CAD build for the part. Positions are in the model's coordinates, mm. A direction names the side the tool comes from. Give positions to 0.01 mm unless a question says otherwise; leave off trailing zeros. Write each loop counter-clockwise with the first axis right and the second up, starting at its lowest first coordinate (ties: lowest second). Pieces come first, ordered by that corner, then holes. Notation, with made-up numbers: (12, 31) - (24, 31) arc R20 ccw to (24, 64) - close; hole circle Ø6 at (-10.5, 73). An arc over 180 degrees is marked (long way). Answer as a JSON object with one key per item and string values.
from build123d import *

# Parameters (mm, degrees)
SKETCH1_W                                     = 80
SKETCH1_H                                     = 80
BOSS_EXTRUDE1_DEPTH                           = 23.7
CUT_EXTRUDE1_DEPTH                            = 1
SKETCH3_W                                     = 15
SKETCH3_H                                     = 15
CUT_EXTRUDE2_DEPTH                            = 95.785112281
SKETCH4_W                                     = 60
SKETCH4_H                                     = 13.7
CUT_EXTRUDE3_DEPTH                            = 114.918214427
SKETCH5_R                                     = 3
SKETCH5_R_2                                   = 2
CUT_EXTRUDE4_DEPTH                            = 114.918214427
CBORE_FOR_M5_HEX_SOCKET_HEAD_CAP1_D           = 5.5
CBORE_FOR_M5_HEX_SOCKET_HEAD_CAP1_CBORE_D     = 10
CBORE_FOR_M5_HEX_SOCKET_HEAD_CAP1_CBORE_DEPTH = 15
M3X0_5_TAPPED_HOLE1_D                         = 2.5
M2X0_4_TAPPED_HOLE1_REACH                     = 95.041
M2X0_4_TAPPED_HOLE1_BORE_R                    = 0.8


with BuildPart() as part:
    # Sketch1 → Boss-Extrude1 (new body)
    with BuildSketch(Plane(origin=(0, 0, 0), x_dir=(1, 0, 0), z_dir=(0, 1, 0))):
        with Locations((-37.560747664, 9.530373832)):
            Rectangle(SKETCH1_W, SKETCH1_H)
    extrude(amount=BOSS_EXTRUDE1_DEPTH)

    # Sketch2 → Cut-Extrude1 (cut)
    with BuildSketch(Plane(origin=(0, 23.7, 0), x_dir=(1, 0, 0), z_dir=(0, 1, 0))):
        Polygon((2.439252336, -28.669626168), (-22.560747664, -28.669626168), (-22.560747664, -18.669626168), (-32.560747664, -18.669626168), (-32.560747664, -28.669626168), (-67.560747664, -28.669626168), (-67.560747664, 47.730373832), (-32.560747664, 47.730373832), (-32.560747664, 37.730373832), (-22.560747664, 37.730373832), (-22.560747664, 47.730373832), (2.439252336, 47.730373832), align=None)
    extrude(amount=-CUT_EXTRUDE1_DEPTH, mode=Mode.SUBTRACT)

    # Sketch3 → Cut-Extrude2 (cut, through all)
    with BuildSketch(Plane(origin=(0, 22.7, 0), x_dir=(1, 0, 0), z_dir=(0, 1, 0))):
        with Locations((-55.060747664, -16.169626168)):
            Rectangle(SKETCH3_W, SKETCH3_H)
        with Locations((-55.060747664, 5.830373832)):
            Rectangle(SKETCH3_W, SKETCH3_H)
        with Locations((-55.060747664, 27.830373832)):
            Rectangle(SKETCH3_W, SKETCH3_H)
    extrude(amount=-CUT_EXTRUDE2_DEPTH, mode=Mode.SUBTRACT)

    # Sketch4 → Cut-Extrude3 (cut, through all)
    with BuildSketch(Plane.XY.offset(30.469626168)):
        with Locations((-47.560747664, 6.85)):
            Rectangle(SKETCH4_W, SKETCH4_H)
    extrude(amount=-CUT_EXTRUDE3_DEPTH, mode=Mode.SUBTRACT)

    # Sketch5 → Cut-Extrude4 (cut, through all)
    with BuildSketch(Plane.XY.offset(30.469626168)):
        with Locations((-66.560747664, 18.7)):
            Circle(SKETCH5_R)
        with Locations((-44.560747664, 18.7)):
            Circle(SKETCH5_R_2)
    extrude(amount=-CUT_EXTRUDE4_DEPTH, mode=Mode.SUBTRACT)

    # CBORE for M5 Hex Socket Head Cap1 (through all)
    with Locations(Plane(origin=(0, 22.7, 0), x_dir=(1, 0, 0), z_dir=(0, 1, 0))):
        with Locations((-7.560747664, -20.469626168), (-7.560747664, -0.469626168), (-7.560747664, 19.530373832), (-7.560747664, 39.530373832)):
            CounterBoreHole(CBORE_FOR_M5_HEX_SOCKET_HEAD_CAP1_D / 2, CBORE_FOR_M5_HEX_SOCKET_HEAD_CAP1_CBORE_D / 2, CBORE_FOR_M5_HEX_SOCKET_HEAD_CAP1_CBORE_DEPTH)

    # M3x0.5 Tapped Hole1 (through all)
    with Locations(Plane(origin=(0, 23.7, 0), x_dir=(1, 0, 0), z_dir=(0, 1, 0))):
        with Locations((-27.560747664, -23.669626168), (-27.560747664, 42.730373832), (-72.523263375, -23.669626168), (-72.523263375, 42.730373832)):
            Hole(M3X0_5_TAPPED_HOLE1_D / 2)

    # M2x0.4 Tapped Hole1 bore → M2x0.4 Tapped Hole1 (cut, up to next)
    with BuildSketch(Plane(origin=(0, 13.7, 0), x_dir=(-1, 0, 0), z_dir=(0, -1, 0)), mode=Mode.PRIVATE) as m2x0_4_tapped_hole1_sk1:
        with Locations((66.560747664, -15.469626168)):
            Circle(M2X0_4_TAPPED_HOLE1_BORE_R)
    m2x0_4_tapped_hole1_tool1 = extrude(m2x0_4_tapped_hole1_sk1.sketch, amount=-M2X0_4_TAPPED_HOLE1_REACH, mode=Mode.PRIVATE) & part.part
    # M2x0.4 Tapped Hole1 bore → M2x0.4 Tapped Hole1 (cut, up to next)
    with BuildSketch(Plane(origin=(0, 13.7, 0), x_dir=(-1, 0, 0), z_dir=(0, -1, 0)), mode=Mode.PRIVATE) as m2x0_4_tapped_hole1_sk2:
        with Locations((44.560747664, -15.469626168)):
            Circle(M2X0_4_TAPPED_HOLE1_BORE_R)
    m2x0_4_tapped_hole1_tool2 = extrude(m2x0_4_tapped_hole1_sk2.sketch, amount=-M2X0_4_TAPPED_HOLE1_REACH, mode=Mode.PRIVATE) & part.part
    # M2x0.4 Tapped Hole1 bore → M2x0.4 Tapped Hole1 (cut, up to next)
    with BuildSketch(Plane(origin=(0, 13.7, 0), x_dir=(-1, 0, 0), z_dir=(0, -1, 0)), mode=Mode.PRIVATE) as m2x0_4_tapped_hole1_sk3:
        with Locations((66.560747664, 34.530373832)):
            Circle(M2X0_4_TAPPED_HOLE1_BORE_R)
    m2x0_4_tapped_hole1_tool3 = extrude(m2x0_4_tapped_hole1_sk3.sketch, amount=-M2X0_4_TAPPED_HOLE1_REACH, mode=Mode.PRIVATE) & part.part
    # M2x0.4 Tapped Hole1 bore → M2x0.4 Tapped Hole1 (cut, up to next)
    with BuildSketch(Plane(origin=(0, 13.7, 0), x_dir=(-1, 0, 0), z_dir=(0, -1, 0)), mode=Mode.PRIVATE) as m2x0_4_tapped_hole1_sk4:
        with Locations((44.560747664, 34.530373832)):
            Circle(M2X0_4_TAPPED_HOLE1_BORE_R)
    m2x0_4_tapped_hole1_tool4 = extrude(m2x0_4_tapped_hole1_sk4.sketch, amount=-M2X0_4_TAPPED_HOLE1_REACH, mode=Mode.PRIVATE) & part.part
    add(m2x0_4_tapped_hole1_tool1.solids().sort_by_distance((-66.560748, 13.7, 15.469626))[0], mode=Mode.SUBTRACT)
    add(m2x0_4_tapped_hole1_tool2.solids().sort_by_distance((-44.560748, 13.7, 15.469626))[0], mode=Mode.SUBTRACT)
    add(m2x0_4_tapped_hole1_tool3.solids().sort_by_distance((-66.560748, 13.7, -34.530374))[0], mode=Mode.SUBTRACT)
    add(m2x0_4_tapped_hole1_tool4.solids().sort_by_distance((-44.560748, 13.7, -34.530374))[0], mode=Mode.SUBTRACT)


solid = part.part
Item 1: Probe line 1 (Z direction, x = -7.5, y = 14.25); line 2 (Z direction, x = -52, y = 19.5); line 3 (X direction, y = 17, z = -22). List the from-to ranges inside material, lowest first. Write a range as from..to.
Entries:
{"line 1": "-49.53..-44.53, -34.53..-24.53, -14.53..-4.53, 5.47..15.47, 25.47..30.47", "line 2": "-49.53..-35.33, -20.33..-13.33, 1.67..8.67, 23.67..30.47", "line 3": "-77.56..-69.03, -64.09..-62.56, -47.56..-45.61, -43.51..-11.91, -3.21..2.44"}
Item 2: Mould opens along Z. For faces 4 (the flat face through (-8, 0, -10)), 5 (the flat face through (-55, 18, -20.33)), 6 (the flat face through (-29, 14, 30.47)) say: +Z half, -Z half, draft (parallel to the pull), parting line (faces both ways), or undercut.
Entries:
{"face 4": "draft", "face 5": "undercut", "face 6": "+Z half"}
Item 3: Cut at C-C (x = -16.5). Give the cut face in (y, z).
Entries:
{"outline": "(0, -49.53) - (23.7, -49.53) - (23.7, -47.73) - (22.7, -47.73) - (22.7, 28.67) - (23.7, 28.67) - (23.7, 30.47) - (0, 30.47) - close"}
Item 4: Cut at B-B (y = 18.7). State how many separate pieces and enclosed holes the cut face has, and give its area (3 significant figures).
Entries:
{"separate pieces": "3", "enclosed holes": "11", "area": "4,590 mm2"}
Item 5: Which spindle directions (+Z, -Z, +X, -X, +Y, -Y) get a long thin tool onto all of the face, cutting with end or side? Do faces 1 (the flat face through (-47.561, 18, -6)), 2 (the flat face through (-41, 13.7, -9)), 3 (the flat face through (-5, 7.7, -17)). Say none if no direction does.
Entries:
{"face 1": "+Y, -Y", "face 2": "+Z, -Z, -X, -Y", "face 3": "+Y"}
Item 6: Flat gauge pins, fed straight in: P1, Ø5, axis at x = -6, z = -17, coming from the +Y side; P2, Ø8, axis at x = -7.56, z = -19.53, coming from the +Y side; P3, Ø0.8, axis at y = 23.5, z = 25.5, coming from the +X side; P4, Ø4.5, axis at x = -7.56, z = -19.53, coming from the -Y side. Where does each tip first touch, or does it go through?
Entries:
{"P1": "y = 22.7", "P2": "y = 7.7", "P3": "x = -22.56", "P4": "through"}
Item 7: Cut at D-D (y = 2.25). Give the cut face in (x, z).
Entries:
{"outline": "(-17.56, -49.53) - (2.44, -49.53) - (2.44, 30.47) - (-17.56, 30.47) - close; hole circle Ø5.5 at (-7.56, -39.53); hole circle Ø5.5 at (-7.56, -19.53); hole circle Ø5.5 at (-7.56, 0.47); hole circle Ø5.5 at (-7.56, 20.47)"}
Item 8: Cut at A-A (z = 12). Give the cut face in (x, y), and give its area (3 significant figures).
Entries:
{"outline": "(-77.56, 13.7) - (-62.56, 13.7) - (-62.56, 22.7) - (-67.56, 22.7) - (-67.56, 23.7) - (-77.56, 23.7) - close; (-47.56, 13.7) - (-17.56, 13.7) - (-17.56, 0) - (2.44, 0) - (2.44, 22.7) - (-47.56, 22.7) - close; hole circle Ø6 at (-66.56, 18.7); hole circle Ø4 at (-44.56, 18.7)", "area": "828 mm2"}
